from build123d import *

# Parameters (mm, degrees)
F0_W     = 81.3
F0_H     = 13
F0_R     = 2.4
F1_DEPTH = 6.5
F2_R     = 5.5
F3_W     = 1
F3_H     = 2.5
F4_DEPTH = 5
F5_W     = 1
F5_H     = 2.5
F6_DEPTH = 5


with BuildPart() as f1:
    # F0 (on Top) → F1 (new body)
    with BuildSketch(Plane.XY):
        with Locations((0, 2.616273)):
            Rectangle(F0_W, F0_H)
        with Locations((-33.75, 2.616273)):
            Circle(F0_R, mode=Mode.SUBTRACT)
        with Locations((33.75, 2.616273)):
            Circle(F0_R, mode=Mode.SUBTRACT)
    extrude(amount=F1_DEPTH)

    # F2
    f2_edges = [f1.edges().sort_by_distance(p)[0] for p in [
        (-40.65, 9.116273, 3.25),
        (-40.65, -3.883727, 3.25),
        (40.65, -3.883727, 3.25),
        (40.65, 9.116273, 3.25),
    ]]
    fillet(f2_edges, radius=F2_R)

    # F3 (on face) → F4 (join)
    with BuildSketch(Plane.XZ.offset(3.883727)):
        with Locations((25.7837, 1.25)):
            Rectangle(F3_W, F3_H)
    extrude(amount=F4_DEPTH)

    # F5 (on face) → F6 (join)
    with BuildSketch(Plane(origin=(0, 9.116273, 0), x_dir=(-1, 0, 0), z_dir=(0, 1, 0))):
        with Locations((25.072782, 1.25)):
            Rectangle(F5_W, F5_H)
    extrude(amount=F6_DEPTH)


solid = f1.part
CAD build for the part. Positions are in the model's coordinates, mm. A direction names the side the tool comes from. Round coordinates to 2 decimals unless told otherwise and drop trailing zeros. Order: outer loops, then holes, each group sorted by start corner. A loop starts at its lowest first (then second) coordinate and runs counter-clockwise, first axis right, second up. Notation, with made-up numbers: (83, -4) -> (94, -4) arc R22 cw to (94, 20) -> close; hole circle Ø11 at (-1, 26). An arc over 180 degrees is marked (long way). Write item = value, one per line. Start each with the question number.
(1) Cut at C-C, the plane y = 11.5. List the corners of the cut face in (x, z), then the cut area to 3 significant figures.
(2) Cut at A-A, the plane x = 33.75. List the corners of the cut face in (y, z), then the cut area to 3 significant figures.
(3) Pin check, flat tips, straight feed: P1, Ø3, axis at y = -7, z = 1.5, coming from the +X side; P2, Ø3, axis at y = 12.5, z = 1.5, coming from the -X side; P3, Ø2, axis at x = -13.5, z = 4, coming from the +Y side; P4, Ø7.5, axis at x = 33.75, y = 2.62, coming from the -Z side. Stop position of each tip, or through.
(4) Probe line 1 (Y direction, x = -33.75, z = 5); line 2 (X direction, y = -6.75, z = 2.25); line 3 (Y direction, x = -10, z = 2). List the from-to ranges inside material, lowest first. Write a range as [from, to].
(5) Which spindle directions (+Z, -Z, +X, -X, +Y, -Y) get a long thin tool onto all of the face, cutting with end or side? Do faces 4 (the flat face through (-24.573, 12, 1)), 5 (the flat face through (-25.573, 12, 1)), 6 (the flat face through (26.284, -6, 1)). Say none if no direction does.
(6) Cut at B-B, the plane z = 1.5. List the corners of the cut face in (x, y).
(7) Cut at D-D, the plane x = -19. List the corners of the cut face in (y, z), then the cut area to 3 significant figures.
(8) Pull direction X, two halves, no side cores. Call faces 1 (the flat face through (40.65, 3, 3)), 2 (the cylindrical face through (-35.655, 1.156, 3.204)), 3 (the cylindrical face through (-39.08, -2.23, 3.3)): released by +X, released by -X, zero draft, split by the parting line, or undercut.
Model answer:
q1.outline = (-25.57, 0) -> (-24.57, 0) -> (-24.57, 2.5) -> (-25.57, 2.5) -> close
q1.area = 2.50 mm2
q2.outline = (-3.88, 0) -> (0.22, 0) -> (0.22, 6.5) -> (-3.88, 6.5) -> close; (5.02, 0) -> (9.12, 0) -> (9.12, 6.5) -> (5.02, 6.5) -> close
q2.area = 53.3 mm2
q3.P1 = 26.28
q3.P2 = -25.57
q3.P3 = 9.12
q3.P4 = 0
q4.line_1 = [-3.88, 0.22], [5.02, 9.12]
q4.line_2 = [25.28, 26.28]
q4.line_3 = [-3.88, 9.12]
q5.face_4 = +Z, -Z, +X, +Y
q5.face_5 = +Z, -Z, -X, +Y
q5.face_6 = +Z, -Z, +X, -Y
q6.outline = (-40.65, 1.62) arc R5.5 ccw to (-35.15, -3.88) -> (25.28, -3.88) -> (25.28, -8.88) -> (26.28, -8.88) -> (26.28, -3.88) -> (35.15, -3.88) arc R5.5 ccw to (40.65, 1.62) -> (40.65, 3.62) arc R5.5 ccw to (35.15, 9.12) -> (-24.57, 9.12) -> (-24.57, 14.12) -> (-25.57, 14.12) -> (-25.57, 9.12) -> (-35.15, 9.12) arc R5.5 ccw to (-40.65, 3.62) -> close; hole circle Ø4.8 at (-33.75, 2.62); hole circle Ø4.8 at (33.75, 2.62)
q7.outline = (-3.88, 0) -> (9.12, 0) -> (9.12, 6.5) -> (-3.88, 6.5) -> close
q7.area = 84.5 mm2
q8.face_1 = released by +X
q8.face_2 = undercut
q8.face_3 = released by -X
